from build123d import *

# Parameters (mm, degrees)
F0_R     = 4
F1_DEPTH = 7
F4_D     = 4.2


with BuildPart() as f1:
    # F0 (on Right) → F1 (new body, symmetric)
    with BuildSketch(Plane.YZ):
        Polygon((-21, 0), (0, 0), (21, 0), (21, 6), (9, 6), (9, 33), (0, 33), (-9, 33), (-9, 6), (-21, 6), align=None)
        with Locations((0, 20)):
            Circle(F0_R, mode=Mode.SUBTRACT)
    extrude(amount=F1_DEPTH, both=True)

    # F4 (through all)
    with Locations(Plane.XY.offset(6)):
        with Locations((0, -16), (0, 16)):
            Hole(F4_D / 2)


solid = f1.part
Model file for the job. Use its own axes, mm. A direction names the side the tool comes from. Give positions to 0.01 mm unless a question says otherwise; leave off trailing zeros. Order: outer loops, then holes, each group sorted by start corner. A loop starts at its lowest first (then second) coordinate and runs counter-clockwise, first axis right, second up. Notation, with made-up numbers: (85.25, 79) - (102.25, 79) arc R30 ccw to (102.25, 109) - close; hole circle Ø2 at (-32, -15.5). An arc over 180 degrees is marked (long way). Write item = value, one per line. Start each with the question number.
1. Probe line 1 along Y through (x, z) = (0, 4); line 2 along Z through (x, y) = (-0.5, 0); line 3 along Z through (x, y) = (2.75, -13). List the from-to ranges inside material, lowest first.
2. Cut at A-A, the plane x = 0. List the corners of the cut face in (y, z), and give its area (3 significant figures).
3. Cut at D-D, the plane x = 4. List the corners of the cut face in (y, z).
4. Two-plate mould, pull along X, no slides. Class faces 4 (the flat face through (0.1, -13.6, 6)), 5 (the cylindrical face through (0.273, -13.918, 2.958)), 6 (the flat face through (7, 0, 13)): pulls with the +X half, pulls with the -X half, needs draft (parallel to the pull), parting line crosses it, or undercut.
5. Cut at B-B, the plane z = 20. List the corners of the cut face in (x, y).
6. Which spindle directions (+Z, -Z, +X, -X, +Y, -Y) get a long thin tool onto all of the face, cutting with end or side? Do faces 1 (the flat face through (0, -9, 20)), 2 (the cylindrical face through (-0.098, -0.521, 23.966)), 3 (the flat face through (0.1, 13.75, 6)). Say none if no direction does.
7. Drop flat-ended pins along their axis: P1, Ø6, axis at x = 1.5, z = 20, coming from the -Y side; P2, Ø2.5, axis at x = 0, y = 16, coming from the +Z side; P3, Ø1.5, axis at x = -5, z = 20.5, coming from the +Y side; P4, Ø6, axis at x = 1.5, y = 12.5, coming from the +Z side. Give the stop position or say it passes through.
8. Cut at C-C, the plane y = 16. List the corners of the cut face in (x, z).
Taken from the geometry:
q1.line_1 = -21 to -18.1, -13.9 to 13.9, 18.1 to 21
q1.line_2 = 0 to 16, 24 to 33
q1.line_3 = 0 to 6
q2.outline = (-21, 0) - (-18.1, 0) - (-18.1, 6) - (-21, 6) - close; (-13.9, 0) - (13.9, 0) - (13.9, 6) - (9, 6) - (9, 33) - (-9, 33) - (-9, 6) - (-13.9, 6) - close; (18.1, 0) - (21, 0) - (21, 6) - (18.1, 6) - close; hole circle Ø8 at (0, 20)
q2.area = 637 mm²
q3.outline = (-21, 0) - (21, 0) - (21, 6) - (9, 6) - (9, 33) - (-9, 33) - (-9, 6) - (-21, 6) - close; hole circle Ø8 at (0, 20)
q4.face_4 = needs draft
q4.face_5 = undercut
q4.face_6 = pulls with the +X half
q5.outline = (-7, -9) - (7, -9) - (7, -4) - (-7, -4) - close; (-7, 4) - (7, 4) - (7, 9) - (-7, 9) - close
q6.face_1 = +Z, +X, -X, -Y
q6.face_2 = +X, -X
q6.face_3 = +Z, +X, -X, +Y
q7.P1 = -9
q7.P2 = through
q7.P3 = 9
q7.P4 = 6
q8.outline = (-7, 0) - (-2.1, 0) - (-2.1, 6) - (-7, 6) - close; (2.1, 0) - (7, 0) - (7, 6) - (2.1, 6) - close
